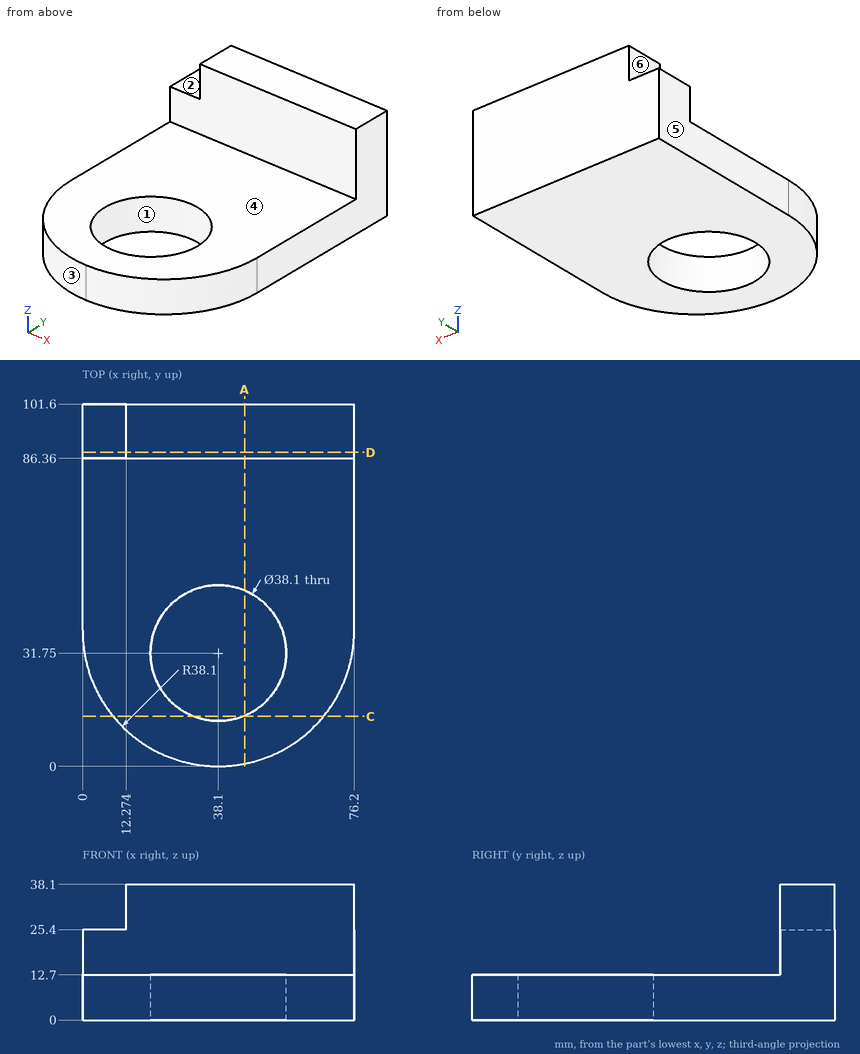
Input: dimensioned drawing with shaded views. Units: mm. Origin: part minimum x, y, z. A direction names the side the tool comes from. Give positions to 0.01 mm unless a question says otherwise; leave off trailing zeros. Write each loop counter-clockwise with the first axis right and the second up, starting at its lowest first coordinate (ties: lowest second). Pieces come first, ordered by that corner, then holes.
Q1. Section A-A, the plane x = 45.5. Output: boundary loops of the cut face in (y, z), plus the area to 3 significant figures.
Q2. Set-up query: the marked faces 4, 5 and 6. Return all of +Z, -Z, +X, -X, +Y, -Y with unobstructed straight access to the full face (end or side cutting, diameter ignored); none if empty.
Q3. First-contact query: P1, Ø10, axis at y = 97, z = 34.5, coming from the -X side; P2, Ø20.5, axis at x = 22.5, z = 31.5, coming from the -Y side; P3, Ø1, axis at x = 56.5, z = 5.5, coming from the -Y side. Flat tips, straight axial feed; report the tip coordinate or a pass-through.
Q4. Section D-D, the plane y = 88. Output: boundary loops of the cut face in (x, z).
Q5. Section C-C, the plane y = 14. Output: boundary loops of the cut face in (x, z).
Q6. Material intervals for probe 1 along Y at (x, z) = (38.1, 9.75); probe 2 along Z at (x, y) = (60, 35.5); probe 3 along X at (y, z) = (31, 3) (1 decimal), sorted ascending.
Q7. Pull-direction query (Y, two-part tool) for the marked faces 1, 2 and 3; classes: pulls with the +Y half, pulls with the -Y half, needs draft (parallel to the pull), parting line crosses it, or undercut.
Filled in:
1. outline: (0.73, 0) - (14.2, 0) - (14.2, 12.7) - (0.73, 12.7) - close; (49.3, 0) - (101.6, 0) - (101.6, 38.1) - (86.36, 38.1) - (86.36, 12.7) - (49.3, 12.7) - close
1. area: 1,220 mm2
2. face 4: +Z, +X, -X, -Y
2. face 5: +Z, -Z, -X, +Y, -Y
2. face 6: +Z, -X, +Y, -Y
3. P1: stops at x = 12.27
3. P2: stops at y = 86.36
3. P3: stops at y = 4.47
4. outline: (0, 0) - (76.2, 0) - (76.2, 38.1) - (12.27, 38.1) - (12.27, 25.4) - (0, 25.4) - close
5. outline: (8.59, 0) - (31.18, 0) - (31.18, 12.7) - (8.59, 12.7) - close; (45.02, 0) - (67.61, 0) - (67.61, 12.7) - (45.02, 12.7) - close
6. probe 1: y = 0 to 12.7, 50.8 to 101.6
6. probe 2: z = 0 to 12.7
6. probe 3: x = 0.7 to 19.1, 57.1 to 75.5
7. face 1: undercut
7. face 2: needs draft
7. face 3: pulls with the -Y half
